The model under review builds one solid part; all positions refer to its coordinate system, in mm. A direction names the side the tool comes from. Round coordinates to 2 decimals unless told otherwise and drop trailing zeros. Order: outer loops, then holes, each group sorted by start corner. A loop starts at its lowest first (then second) coordinate and runs counter-clockwise, first axis right, second up. Notation, with made-up numbers: M 22.5,-11 L 64.5,-11 A20 cw 64.5,0 Z; hole C 9.5,-14.5 d5. An arc over 180 degrees is marked long. Use a Markdown table: item, result. Add a question column.
1. Consider section B-B on y = 0. State the section outline as (x, z) points.
2. For faces 4 (the cylindrical face through (-1.2, 33.7, 9.9)), 5 (the cylindrical face through (-5, 0, -25)), 6 (the cylindrical face through (5, 0, -25)), list the 3-axis set-ups (+Z, -Z, +X, -X, +Y, -Y) from which the entire face can be reached by the end or side of a thin tool; tool diameter is ignored.
3. Insertion check: P1, Ø10, axis at x = 2.5, y = -26, coming from the +Z side; P2, Ø12, axis at x = 25.5, z = 10, coming from the +Y side; P3, Ø6, axis at x = -26, z = 5, coming from the +Y side; P4, Ø0.5, axis at x = 0, z = -30.5, coming from the +Y side. Each pin has a flat end and moves straight along its axis. Give the tip position at first contact, or say it passes through.
4. The part is to be moulded in two halves that separate along Y. For faces 1 (the flat face through (0, 35, 20)), 2 (the cylindrical face through (-18.952, -28.566, 9.86)), 3 (the cylindrical face through (-37.64, -15.61, -4.93)), say which applies: +Y half, -Y half, draft (parallel to the pull), parting line (faces both ways), or undercut.
5. Consider section A-A on z = 12. Count the separate pieces of the cut face and the enclosed holes in it, then the cut area to 3 significant figures.
6. To check wall thickness, follow probe 1 along X at (y, z) = (-28, 0.5); probe 2 along Z at (x, y) = (-7, -16); probe 3 along Z at (x, y) = (-2, -2). State the ranges of each line that lie inside material, in increasing order.
7. Consider section D-D on x = 12. State the section outline as (y, z) points.
from build123d import *

# Parameters (mm, degrees)
SKETCH1_R              = 1.5
BOSS_EXTRUDE1_DEPTH    = 20
BOSS_EXTRUDE1_2_DEPTH  = 20
BOSS_EXTRUDE1_3_DEPTH  = 20
BOSS_EXTRUDE1_4_DEPTH  = 20
BOSS_EXTRUDE1_5_DEPTH  = 20
BOSS_EXTRUDE1_6_DEPTH  = 20
BOSS_EXTRUDE1_7_DEPTH  = 20
BOSS_EXTRUDE1_8_DEPTH  = 20
BOSS_EXTRUDE1_9_DEPTH  = 20
BOSS_EXTRUDE1_10_DEPTH = 20
SKETCH2_R              = 40.75
BOSS_EXTRUDE2_DEPTH    = 10
SKETCH3_R              = 5
BOSS_EXTRUDE3_DEPTH    = 30
SKETCH4_W              = 1
SKETCH4_H              = 2
BOSS_EXTRUDE4_DEPTH    = 30


with BuildPart() as part:
    # Sketch1 → Boss-Extrude1 (new body)
    with BuildSketch(Plane.XY):
        with Locations((0, 34.6)):
            Circle(SKETCH1_R)
    extrude(amount=BOSS_EXTRUDE1_DEPTH)



with BuildPart() as body_2:
    # Sketch1 → Boss-Extrude1 2 (new body)
    with BuildSketch(Plane.XY):
        with Locations((20.337369729, 27.991988005)):
            Circle(SKETCH1_R)
    extrude(amount=BOSS_EXTRUDE1_2_DEPTH)


with BuildPart() as body_3:
    # Sketch1 → Boss-Extrude1 3 (new body)
    with BuildSketch(Plane.XY):
        with Locations((32.906555464, 10.691988005)):
            Circle(SKETCH1_R)
    extrude(amount=BOSS_EXTRUDE1_3_DEPTH)


with BuildPart() as body_4:
    # Sketch1 → Boss-Extrude1 4 (new body)
    with BuildSketch(Plane.XY):
        with Locations((32.906555464, -10.691988005)):
            Circle(SKETCH1_R)
    extrude(amount=BOSS_EXTRUDE1_4_DEPTH)


with BuildPart() as body_5:
    # Sketch1 → Boss-Extrude1 5 (new body)
    with BuildSketch(Plane.XY):
        with Locations((20.337369729, -27.991988005)):
            Circle(SKETCH1_R)
    extrude(amount=BOSS_EXTRUDE1_5_DEPTH)


with BuildPart() as body_6:
    # Sketch1 → Boss-Extrude1 6 (new body)
    with BuildSketch(Plane.XY):
        with Locations((0, -34.6)):
            Circle(SKETCH1_R)
    extrude(amount=BOSS_EXTRUDE1_6_DEPTH)


with BuildPart() as body_7:
    # Sketch1 → Boss-Extrude1 7 (new body)
    with BuildSketch(Plane.XY):
        with Locations((-20.337369729, -27.991988005)):
            Circle(SKETCH1_R)
    extrude(amount=BOSS_EXTRUDE1_7_DEPTH)


with BuildPart() as body_8:
    # Sketch1 → Boss-Extrude1 8 (new body)
    with BuildSketch(Plane.XY):
        with Locations((-32.906555464, -10.691988005)):
            Circle(SKETCH1_R)
    extrude(amount=BOSS_EXTRUDE1_8_DEPTH)


with BuildPart() as body_9:
    # Sketch1 → Boss-Extrude1 9 (new body)
    with BuildSketch(Plane.XY):
        with Locations((-32.906555464, 10.691988005)):
            Circle(SKETCH1_R)
    extrude(amount=BOSS_EXTRUDE1_9_DEPTH)


with BuildPart() as body_10:
    # Sketch1 → Boss-Extrude1 10 (new body)
    with BuildSketch(Plane.XY):
        with Locations((-20.337369729, 27.991988005)):
            Circle(SKETCH1_R)
    extrude(amount=BOSS_EXTRUDE1_10_DEPTH)


with BuildPart() as part_1:
    add(part.part)

    add(body_2.part)  # Boss-Extrude2 merges body 2

    add(body_3.part)  # Boss-Extrude2 merges body 3

    add(body_4.part)  # Boss-Extrude2 merges body 4

    add(body_5.part)  # Boss-Extrude2 merges body 5

    add(body_6.part)  # Boss-Extrude2 merges body 6

    add(body_7.part)  # Boss-Extrude2 merges body 7

    add(body_8.part)  # Boss-Extrude2 merges body 8

    add(body_9.part)  # Boss-Extrude2 merges body 9

    add(body_10.part)  # Boss-Extrude2 merges body 10
    # Sketch2 → Boss-Extrude2 (add)
    with BuildSketch(Plane(origin=(0, 0, 0), x_dir=(-1, 0, 0), z_dir=(0, 0, -1))):
        Circle(SKETCH2_R)
    extrude(amount=BOSS_EXTRUDE2_DEPTH)

    # Sketch3 → Boss-Extrude3 (add)
    with BuildSketch(Plane(origin=(0, 0, -10), x_dir=(-1, 0, 0), z_dir=(0, 0, -1))):
        Circle(SKETCH3_R)
    extrude(amount=BOSS_EXTRUDE3_DEPTH)

    # Sketch4 → Boss-Extrude4 (add)
    with BuildSketch(Plane(origin=(0, 0, -40), x_dir=(-1, 0, 0), z_dir=(0, 0, -1))):
        with Locations((0, 5.5)):
            Rectangle(SKETCH4_W, SKETCH4_H)
        with Locations((0, -5.5)):
            Rectangle(SKETCH4_W, SKETCH4_H)
    extrude(amount=-BOSS_EXTRUDE4_DEPTH)


solid = part_1.part
Answer block:
| question | item | result |
|---|---|---|
| 1 | outline | M -40.75,-10 L -5,-10 L -5,-40 L 5,-40 L 5,-10 L 40.75,-10 L 40.75,0 L -40.75,0 Z |
| 2 | face 4 | +Z |
| 2 | face 5 | -Z, -X |
| 2 | face 6 | -Z, +X |
| 3 | P1 | z = 0 |
| 3 | P2 | y = 29.49 |
| 3 | P3 | through |
| 3 | P4 | y = 6.5 |
| 4 | face 1 | draft |
| 4 | face 2 | undercut |
| 4 | face 3 | parting line |
| 5 | separate pieces | 10 |
| 5 | enclosed holes | 0 |
| 5 | area | 70.7 mm^2 |
| 6 | probe 1 | -21.84 to -18.84, 18.84 to 21.84 |
| 6 | probe 2 | -10 to 0 |
| 6 | probe 3 | -40 to 0 |
| 7 | outline | M -38.94,-10 L 38.94,-10 L 38.94,0 L -38.94,0 Z |
